Source: CAD feature listing. Evaluate the final solid. Frame: model axes, mm. Give positions to 0.01 mm unless a question says otherwise; leave off trailing zeros. Order: outer loops, then holes, each group sorted by start corner. A loop starts at its lowest first (then second) coordinate and runs counter-clockwise, first axis right, second up. Notation, with made-up numbers: M 10,-12.5 L 64,-12.5 A13 ccw 64,-5.5 Z; hole C 31.25,-39 d3. An arc over 180 degrees is marked long. Answer in a Markdown table with one row per item. Add a question column.
(1) Pin query (flat end, axial travel): P1, Ø1.6, axis at x = 24, y = 0, coming from the -Z side; P2, Ø1, axis at y = 12.5, z = 1, coming from the +X side. Return the tip coordinate at first contact, or that it passes through.
(2) Section query C-C, the plane z = 0.85. Count the separate pieces of the cut face and the enclosed holes in it, plus the area to 3 significant figures.
(3) Section query B-B, the plane y = -5. Return loops of the section in (x, z).
(4) Material intervals for line 1 along Y through (x, z) = (-11.5, 1.6); line 2 along X through (y, z) = (24, 0.95); line 3 along Y through (x, z) = (-12, 0.65), sorted ascending.
(5) Section query A-A, the plane x = 8. Return loops of the section in (y, z), plus the area to 3 significant figures.
(6) Mould query, pull axis Y, two halves, no side actions, for faces 1 (the face through (47.69, 15.02, 0.99)), 2 (the face through (-3.47, -15.62, 0.99)), 3 (the face through (-12, 12, 0)). Classes: pulls with the +Y half, pulls with the -Y half, needs draft (parallel to the pull), parting line crosses it, or undercut.
(7) Section query D-D, the plane y = 20. Return loops of the section in (x, z).
from build123d import *

# Parameters (mm, degrees)
SKETCH_R           = 50
SKETCH_R_2         = 16
PAD_DEPTH          = 2
SKETCH001_R        = 1
POCKET_DEPTH       = 282.871995
POCKET_DEPTH_BACK  = 284.871995
POLARPATTERN_COUNT = 8


with BuildPart() as part:
    # Sketch → Pad (new body)
    with BuildSketch(Plane.XY):
        Circle(SKETCH_R)
        Circle(SKETCH_R_2, mode=Mode.SUBTRACT)
    extrude(amount=PAD_DEPTH)

    # Sketch001 → Pocket (cut, two sides)
    with BuildSketch(Plane.XY) as pocket_sk:
        with Locations((24, 0)):
            Circle(SKETCH001_R)
        with Locations((42, 0)):
            Circle(SKETCH001_R)
    pocket = extrude(amount=-POCKET_DEPTH, mode=Mode.SUBTRACT) + extrude(pocket_sk.sketch, amount=POCKET_DEPTH_BACK, mode=Mode.SUBTRACT)

    # PolarPattern: Pocket ×8 about axis
    polarpattern_axis = Axis((0, 0, 0), (0, 0, 1))
    for i in range(1, POLARPATTERN_COUNT):
        add(pocket.rotate(polarpattern_axis, i * 360 / POLARPATTERN_COUNT), mode=Mode.SUBTRACT)


solid = part.part
Values follow:
| question | item | result |
|---|---|---|
| 1 | P1 | passes through |
| 1 | P2 | stops at x = 48.54 |
| 2 | separate pieces | 1 |
| 2 | enclosed holes | 17 |
| 2 | area | 7,000 mm² |
| 3 | outline | M -49.75,0 L -15.2,0 L -15.2,2 L -49.75,2 Z; M 15.2,0 L 49.75,0 L 49.75,2 L 15.2,2 Z |
| 4 | line 1 | y = -48.66 to -11.12, 11.12 to 48.66 |
| 4 | line 2 | x = -43.86 to -1, 1 to 43.86 |
| 4 | line 3 | y = -48.54 to -10.58, 10.58 to 48.54 |
| 5 | outline | M -49.36,0 L -13.86,0 L -13.86,2 L -49.36,2 Z; M 13.86,0 L 49.36,0 L 49.36,2 L 13.86,2 Z |
| 5 | area | 142 mm² |
| 6 | face 1 | parting line crosses it |
| 6 | face 2 | undercut |
| 6 | face 3 | needs draft |
| 7 | outline | M -45.83,0 L 45.83,0 L 45.83,2 L -45.83,2 Z |
